Check sheet for the modelled part. Datum: model origin and axes. Units: mm. A direction names the side the tool comes from. Round coordinates to 2 decimals unless told otherwise and drop trailing zeros. Order: outer loops, then holes, each group sorted by start corner. A loop starts at its lowest first (then second) coordinate and runs counter-clockwise, first axis right, second up. Notation, with made-up numbers: (27.5, 3) -> (41.5, 3) arc R35 ccw to (41.5, 39) -> close; hole circle Ø7 at (-16.5, -30.75). An arc over 180 degrees is marked (long way). Answer in a Markdown table with one row per item.
```python
from build123d import *

# Parameters (mm, degrees)
SKETCH1_W             = 3.683
SKETCH1_H             = 12.7
BOSS_EXTRUDE1_DEPTH   = 22.86
BOSS_EXTRUDE1_2_DEPTH = 22.86
BOSS_EXTRUDE1_3_DEPTH = 22.86
SKETCH2_R             = 1.5875
BOSS_EXTRUDE2_DEPTH   = 3.175
FILLET1_R             = 0.508
SKETCH3_R             = 1.143
CUT_EXTRUDE1_DEPTH    = 12.7
SKETCH4_W             = 12.192
SKETCH4_H             = 3.175
BOSS_EXTRUDE3_DEPTH   = 5.08
FILLET2_R             = 1.5875


with BuildPart() as part:
    # Sketch1 → Boss-Extrude1 (new body)
    with BuildSketch(Plane(origin=(0, 0, 0), x_dir=(1, 0, 0), z_dir=(0, 1, 0))):
        Rectangle(SKETCH1_W, SKETCH1_H)
    extrude(amount=BOSS_EXTRUDE1_DEPTH)



with BuildPart() as body_2:
    # Sketch1 → Boss-Extrude1 2 (new body)
    with BuildSketch(Plane(origin=(0, 0, 0), x_dir=(1, 0, 0), z_dir=(0, 1, 0))):
        with Locations((-15.875, 0)):
            Rectangle(SKETCH1_W, SKETCH1_H)
    extrude(amount=BOSS_EXTRUDE1_2_DEPTH)


with BuildPart() as body_3:
    # Sketch1 → Boss-Extrude1 3 (new body)
    with BuildSketch(Plane(origin=(0, 0, 0), x_dir=(1, 0, 0), z_dir=(0, 1, 0))):
        with Locations((15.875, 0)):
            Rectangle(SKETCH1_W, SKETCH1_H)
    extrude(amount=BOSS_EXTRUDE1_3_DEPTH)


with BuildPart() as part_1:
    add(part.part)

    add(body_2.part)  # Boss-Extrude2 merges body 2

    add(body_3.part)  # Boss-Extrude2 merges body 3
    # Sketch2 → Boss-Extrude2 (add)
    with BuildSketch(Plane(origin=(0, 0, 0), x_dir=(1, 0, 0), z_dir=(0, 1, 0))):
        with BuildLine():
            Line((-23.839553388, -2.733832906), (-17.7165, -6.35))
            Line((-17.7165, -6.35), (17.7165, -6.35))
            Line((17.7165, -6.35), (17.7165, 6.35))
            Line((17.7165, 6.35), (-17.7165, 6.35))
            Line((-17.7165, 6.35), (-23.839553388, 2.733832906))
            ThreePointArc((-23.839553388, 2.733832906), (-25.4, 0), (-23.839553388, -2.733832906))
        make_face()
        with Locations(Location((-22.225, 0, 0), (0, 0, 270))):
            Circle(SKETCH2_R, mode=Mode.SUBTRACT)
    boss_extrude2 = extrude(amount=-BOSS_EXTRUDE2_DEPTH)

    # Mirror1: Boss-Extrude2 across plane
    add(boss_extrude2.mirror(Plane(origin=(0, 0, 0), x_dir=(0, 0, 1), z_dir=(1, 0, 0))))

    # Fillet1
    fillet1_edges = [part_1.edges().sort_by_distance(p)[0] for p in [
        (-14.0335, 0, 0),
        (-17.7165, 0, 0),
        (14.0335, 0, 0),
        (-1.8415, 0, 0),
        (17.7165, 0, 0),
        (1.8415, 0, 0),
    ]]
    fillet(fillet1_edges, radius=FILLET1_R)

    # Sketch3 → Cut-Extrude1 (cut)
    with BuildSketch(Plane(origin=(0, 22.86, 0), x_dir=(1, 0, 0), z_dir=(0, 1, 0))):
        with Locations(Location((15.875, 0, 0), (0, 0, 270))):
            Circle(SKETCH3_R)
        with Locations(Location((0, 0, 0), (0, 0, 270))):
            Circle(SKETCH3_R)
        with Locations(Location((-15.875, 0, 0), (0, 0, 270))):
            Circle(SKETCH3_R)
    extrude(amount=-CUT_EXTRUDE1_DEPTH, mode=Mode.SUBTRACT)

    # Sketch4 → Boss-Extrude3 (add)
    with BuildSketch(Plane(origin=(0, 0, -6.35), x_dir=(-1, 0, 0), z_dir=(0, 0, -1))):
        with Locations((-7.9375, -1.5875)):
            Rectangle(SKETCH4_W, SKETCH4_H)
    extrude(amount=BOSS_EXTRUDE3_DEPTH)

    # Fillet2
    fillet2_edges = [part_1.edges().sort_by_distance(p)[0] for p in [
        (1.8415, -1.5875, -6.35),
        (14.0335, -1.5875, -6.35),
    ]]
    fillet(fillet2_edges, radius=FILLET2_R)


solid = part_1.part
```
(1) Scan lines: probe 1 along X at (y, z) = (17.25, 0); probe 2 along X at (y, z) = (-1.3, 0); probe 3 along X at (y, z) = (3, 0.5). Record each from-to range of solid material in increasing order. Write a range as from..to.
Solutions:
| item | result |
|---|---|
| probe 1 | -17.72..-17.02, -14.73..-14.03, -1.84..-1.14, 1.14..1.84, 14.03..14.73, 17.02..17.72 |
| probe 2 | -25.4..-23.81, -20.64..20.64, 23.81..25.4 |
| probe 3 | -17.72..-14.03, -1.84..1.84, 14.03..17.72 |
(2) Draft check along X on faces 6 (the cylindrical face through (-1.014, 16.599, 0.527)), 7 (the cylindrical face through (-25.4, -1.6, 0)), 8 (the flat face through (16, 22.86, -2)). Enter one of: pulls with the +X half, pulls with the -X half, needs draft (parallel to the pull), parting line crosses it, or undercut.
Solutions:
| item | result |
|---|---|
| face 6 | undercut |
| face 7 | pulls with the -X half |
| face 8 | needs draft |
(3) Depth check by flat-ended pin: pin 1 Ø1.5 at (y, z) = (2.5, 0.5) entering from +X; pin 2 Ø1.1 at (x, z) = (0.5, 0) entering from +Y; pin 3 Ø2.5 at (y, z) = (-2, -10) entering from -X; pin 4 Ø1.8 at (x, z) = (-15.5, 0) entering from +Y. Enter the tip coordinate at first touch or a pass-through.
Solutions:
| item | result |
|---|---|
| pin 1 | x = 17.72 |
| pin 2 | y = 10.16 |
| pin 3 | x = 1.84 |
| pin 4 | y = 22.86 |
(4) Section check A-A on y = 16.5. Give the number of separate pieces and of enclosed holes in the cut face, plus the area to 3 significant figures.
Solutions:
| item | result |
|---|---|
| separate pieces | 3 |
| enclosed holes | 3 |
| area | 128 mm^2 |
(5) Section check C-C on z = -4.25. Record the boundary of the cut face in (x, y) (1 decimal).
Solutions:
| item | result |
|---|---|
| outline | (-21.3, -3.2) -> (21.3, -3.2) -> (21.3, 0) -> (18.2, 0) arc R0.5 cw to (17.7, 0.5) -> (17.7, 22.9) -> (14, 22.9) -> (14, 0.5) arc R0.5 cw to (13.5, 0) -> (2.3, 0) arc R0.5 cw to (1.8, 0.5) -> (1.8, 22.9) -> (-1.8, 22.9) -> (-1.8, 0.5) arc R0.5 cw to (-2.3, 0) -> (-13.5, 0) arc R0.5 cw to (-14, 0.5) -> (-14, 22.9) -> (-17.7, 22.9) -> (-17.7, 0.5) arc R0.5 cw to (-18.2, 0) -> (-21.3, 0) -> close |
(6) Tool access check on faces 1 (the flat face through (-14.2, 10, -6.35)), 2 (the flat face through (20, 0, 0)), 3 (the flat face through (-20, 0, 0)), 4 (the flat face through (-1.842, 12, 0)), 5 (the cylindrical face through (16.84, 16.6, 0.61)). Record the directions out of +Z, -Z, +X, -X, +Y, -Y that give a thin tool (end or side, any length) a straight path to the whole face; none if there is none.
Solutions:
| item | result |
|---|---|
| face 1 | -Z, -X, +Y |
| face 2 | +Z, -Z, +X, +Y |
| face 3 | +Z, -Z, -X, +Y |
| face 4 | +Z, -Z, +Y |
| face 5 | +Y |
(7) Section check B-B on y = 4.5. Record the boundary of the cut face in (x, z).
Solutions:
| item | result |
|---|---|
| outline | (-17.72, -6.35) -> (-14.03, -6.35) -> (-14.03, 6.35) -> (-17.72, 6.35) -> close; (-1.84, -6.35) -> (1.84, -6.35) -> (1.84, 6.35) -> (-1.84, 6.35) -> close; (14.03, -6.35) -> (17.72, -6.35) -> (17.72, 6.35) -> (14.03, 6.35) -> close |
